The figure shows three views and two pictorial views of one solid part (mm, origin at its lowest corner). Answer the questions. Coordinates: 2 decimals unless noted, no trailing zeros. Loops run counter-clockwise (first coordinate to the right, second up) from the corner with the lowest first, then second, coordinate; pieces in that order, holes last. Notation, with made-up numbers: (-25.5, -36.5) - (18.5, -36.5) arc R19 ccw to (18.5, 0.5) - close; hole circle Ø10 at (-40, 53). An arc over 180 degrees is marked (long way). Return JSON: item names as keys, results as strings. Group by question number.
1. Section D-D (z = 53.5) is taken. Write down the section's boundary in (x, y).
2. Section C-C (x = 99) is taken. Write down the section's boundary in (y, z).
3. Find the intervals of material crossed by line 1 along Z through (x, y) = (130.5, 2); line 2 along X through (y, z) = (2.9, 78.5); line 3 along Z through (x, y) = (44, 4), in increasing order.
4. Section B-B (y = 3.4) is taken. Write down the section's boundary in (x, z).
5. Each of these flat-tipped pins is pushed along its axis until it touches: P1, Ø1.8, axis at x = 130.5, z = 78.5, coming from the -Y side; P2, Ø1.5, axis at y = 3.5, z = 88.5, coming from the +X side; P3, Ø2.5, axis at y = 2.5, z = 78, coming from the -X side. Where does it stop, or does it pass through?
6. Section A-A (z = 11.5) is taken. Write down the section's boundary in (x, y).
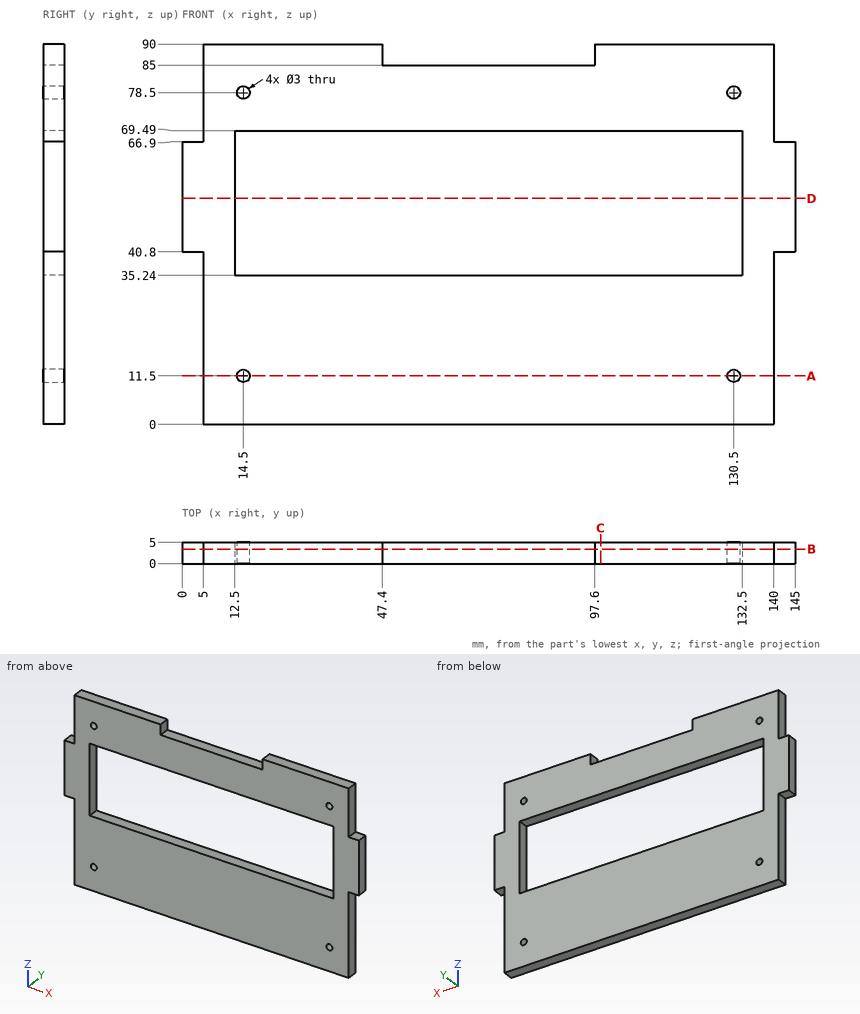
The answers:
{
 "1": {"outline": "(0, 0) - (12.5, 0) - (12.5, 5) - (0, 5) - close; (132.5, 0) - (145, 0) - (145, 5) - (132.5, 5) - close"},
 "2": {"outline": "(0, 0) - (5, 0) - (5, 35.24) - (0, 35.24) - close; (0, 69.49) - (5, 69.49) - (5, 90) - (0, 90) - close"},
 "3": {"line 1": "z = 0 to 10, 13 to 35.24, 69.49 to 77, 80 to 90", "line 2": "x = 5 to 13, 16 to 129, 132 to 140", "line 3": "z = 0 to 35.24, 69.49 to 90"},
 "4": {"outline": "(0, 40.8) - (5, 40.8) - (5, 0) - (140, 0) - (140, 40.8) - (145, 40.8) - (145, 66.9) - (140, 66.9) - (140, 90) - (97.6, 90) - (97.6, 85) - (47.4, 85) - (47.4, 90) - (5, 90) - (5, 66.9) - (0, 66.9) - close; hole (12.5, 35.24) - (132.5, 35.24) - (132.5, 69.49) - (12.5, 69.49) - close; hole circle Ø3 at (14.5, 11.5); hole circle Ø3 at (14.5, 78.5); hole circle Ø3 at (130.5, 11.5); hole circle Ø3 at (130.5, 78.5)"},
 "5": {"P1": "passes through", "P2": "stops at x = 140", "P3": "stops at x = 5"},
 "6": {"outline": "(5, 0) - (13, 0) - (13, 5) - (5, 5) - close; (16, 0) - (129, 0) - (129, 5) - (16, 5) - close; (132, 0) - (140, 0) - (140, 5) - (132, 5) - close"}
}
